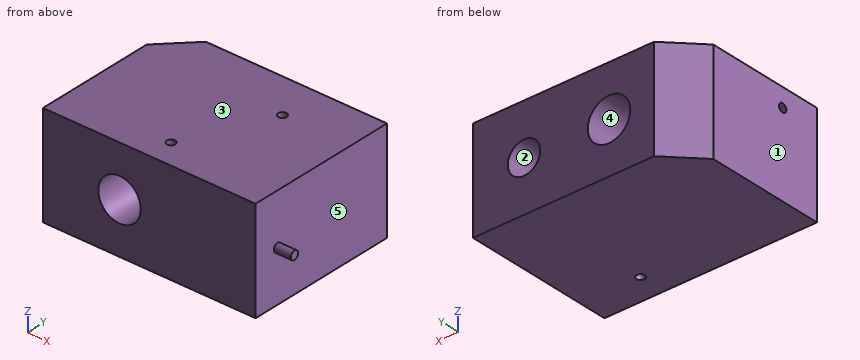
```python
from build123d import *

# Parameters (mm, degrees)
SKETCH1_W                  = 250
SKETCH1_H                  = 180
BOSS_EXTRUDE1_DEPTH        = 120
CUT_EXTRUDE2_DEPTH         = 196.256241898
CUT_EXTRUDE2_DEPTH_BACK    = 120
SKETCH3_R                  = 5
CUT_EXTRUDE3_DEPTH         = 20
SKETCH4_R                  = 5
CUT_EXTRUDE4_DEPTH         = 20
SKETCH6_R                  = 5
CUT_EXTRUDE6_DEPTH         = 20
SKETCH7_R                  = 25
CUT_EXTRUDE7_DEPTH         = 250.849954973
SKETCH5_R                  = 5
BOSS_EXTRUDE2_DEPTH        = 20
F_10_0MM_DOWEL_HOLE1_D     = 10
F_10_0MM_DOWEL_HOLE1_DEPTH = 20
F_10_0MM_DOWEL_HOLE1_TIP   = 3.004303095
SKETCH9_R                  = 19.094825028
CUT_EXTRUDE8_DEPTH         = 50


with BuildPart() as part:
    # Sketch1 → Boss-Extrude1 (new body)
    with BuildSketch(Plane.XY):
        Rectangle(SKETCH1_W, SKETCH1_H)
    extrude(amount=BOSS_EXTRUDE1_DEPTH)

    # Sketch2 → Cut-Extrude2 (cut, two sides: drawn at the far end of the back side and taken through both)
    with BuildSketch(Plane.XY.offset(120).offset(-CUT_EXTRUDE2_DEPTH_BACK)):
        Polygon((320.124564524, 509.15495816), (-88, 90), (-125, 52), (-533.124564524, -367.15495816), (-1371.434480844, 449.094170888), (-518.185351796, 1325.404087208), align=None)
    extrude(amount=CUT_EXTRUDE2_DEPTH + CUT_EXTRUDE2_DEPTH_BACK, mode=Mode.SUBTRACT)

    # Sketch3 → Cut-Extrude3 (cut)
    with BuildSketch(Plane.XY.offset(120)):
        with Locations((45, 40)):
            Circle(SKETCH3_R)
    extrude(amount=-CUT_EXTRUDE3_DEPTH, mode=Mode.SUBTRACT)

    # Sketch4 → Cut-Extrude4 (cut)
    with BuildSketch(Plane.XY.offset(120)):
        with Locations((0, -60)):
            Circle(SKETCH4_R)
    extrude(amount=-CUT_EXTRUDE4_DEPTH, mode=Mode.SUBTRACT)

    # Sketch6 → Cut-Extrude6 (cut)
    with BuildSketch(Plane(origin=(0, 0, 0), x_dir=(-1, 0, 0), z_dir=(0, 0, -1))):
        with Locations((-55, -58)):
            Circle(SKETCH6_R)
    extrude(amount=-CUT_EXTRUDE6_DEPTH, mode=Mode.SUBTRACT)

    # Sketch7 → Cut-Extrude7 (cut, through all)
    with BuildSketch(Plane.XZ.offset(90)):
        with Locations(Location((-35, 60, 0), (0, 0, 270))):
            Circle(SKETCH7_R)
    extrude(amount=-CUT_EXTRUDE7_DEPTH, mode=Mode.SUBTRACT)

    # Sketch5 → Boss-Extrude2 (add)
    with BuildSketch(Plane(origin=(125, 0, 0), x_dir=(0, 0, -1), z_dir=(1, 0, 0))):
        with Locations(Location((-60, -60, 0), (0, 0, 180))):
            Circle(SKETCH5_R)
    extrude(amount=BOSS_EXTRUDE2_DEPTH)

    # Ø10.0mm Dowel Hole1
    with Locations(Plane(origin=(-125, -43, 98), x_dir=(0, 0, -1), z_dir=(-1, 0, 0))):
        with Locations((0, 0)):
            Hole(F_10_0MM_DOWEL_HOLE1_D / 2, depth=F_10_0MM_DOWEL_HOLE1_DEPTH)
            with Locations((0, 0, -(F_10_0MM_DOWEL_HOLE1_DEPTH + F_10_0MM_DOWEL_HOLE1_TIP / 2))):  # 118° drill point
                Cone(0, F_10_0MM_DOWEL_HOLE1_D / 2, F_10_0MM_DOWEL_HOLE1_TIP, mode=Mode.SUBTRACT)

    # Sketch9 → Cut-Extrude8 (cut)
    with BuildSketch(Plane(origin=(0, 90, 0), x_dir=(1, 0, 0), z_dir=(0, 1, 0))):
        with Locations(Location((65, -60, 0), (0, 0, 270))):
            Circle(SKETCH9_R)
    extrude(amount=-CUT_EXTRUDE8_DEPTH, mode=Mode.SUBTRACT)


solid = part.part
```
Geometry check sheet. Reference: the model listing, model coordinates, mm. Face numbers are marked on the shaded views. A direction names the side the tool comes from. Round coordinates to 2 decimals unless told otherwise and drop trailing zeros. Order: outer loops, then holes, each group sorted by start corner. A loop starts at its lowest first (then second) coordinate and runs counter-clockwise, first axis right, second up. Notation, with made-up numbers: (-30, 89.5) - (-15, 89.5) arc R11 ccw to (-15, 96.5) - close; hole circle Ø1 at (88.5, 12.5). An arc over 180 degrees is marked (long way). Use a Markdown table: item, result. Add a question column.
1) Mould release check, pull along Z, two halves, no side actions. Record for the marked faces 3, 4 and 5: released by +Z, released by -Z, zero draft, split by the parting line, or undercut.
2) Section check A-A (x = -35). Record the cut outline in (y, z), then the cut area to 3 significant figures.
3) Thickness scan on line 1 along X through (y, z) = (58.5, 63); line 2 along X through (y, z) = (-27, 60); line 3 along Y through (x, z) = (45, 110.5). Record the ranges inside material, lowest first.
4) Section check C-C (y = 11). Record the cut outline in (x, z), then the cut area to 3 significant figures.
5) Section check B-B (z = 60). Record the cut outline in (x, y).
6) Set-up check for the marked faces 1 and 2: record each of +Z, -Z, +X, -X, +Y, -Y from which the full face is reachable in a straight line by a thin tool's end or side.
7) Section check D-D (x = 65). Record the cut outline in (y, z), then the cut area to 3 significant figures.
8) Gauge pin test, flat ends, axial feed: P1, Ø8, axis at x = 45, y = 40, coming from the +Z side; P2, Ø19, axis at x = 63.5, z = 55, coming from the +Y side; P3, Ø12, axis at x = 42.5, y = -5.5, coming from the -Z side; P4, Ø5, axis at x = 56.5, y = -58, coming from the -Z side. Record the tip position at first contact, or that the pin passes through.
Established:
| question | item | result |
|---|---|---|
| 1 | face 3 | released by +Z |
| 1 | face 4 | undercut |
| 1 | face 5 | zero draft |
| 2 | outline | (-90, 0) - (90, 0) - (90, 35) - (-90, 35) - close; (-90, 85) - (90, 85) - (90, 120) - (-90, 120) - close |
| 2 | area | 12,600 mm2 |
| 3 | line 1 | -118.67 to -59.82, -10.18 to 46.14, 83.86 to 125 |
| 3 | line 2 | -125 to -60, -10 to 125 |
| 3 | line 3 | -90 to 35, 45 to 90 |
| 4 | outline | (-125, 0) - (125, 0) - (125, 120) - (-125, 120) - close; hole circle Ø50 at (-35, 60) |
| 4 | area | 28,000 mm2 |
| 5 | outline | (-125, -90) - (-60, -90) - (-60, 90) - (-88, 90) - (-125, 52) - close; (-10, -90) - (125, -90) - (125, -65) - (145, -65) - (145, -55) - (125, -55) - (125, 90) - (84.09, 90) - (84.09, 40) - (45.91, 40) - (45.91, 90) - (-10, 90) - close |
| 6 | face 1 | +Z, -Z, -X, +Y, -Y |
| 6 | face 2 | +Y |
| 7 | outline | (-90, 0) - (90, 0) - (90, 40.91) - (40, 40.91) - (40, 79.09) - (90, 79.09) - (90, 120) - (-90, 120) - close |
| 7 | area | 19,700 mm2 |
| 8 | P1 | z = 100 |
| 8 | P2 | y = 40 |
| 8 | P3 | z = 0 |
| 8 | P4 | z = 20 |
